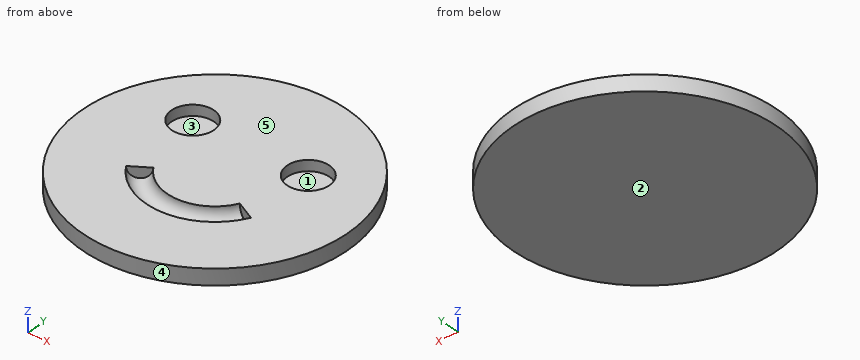
```python
from build123d import *

# Parameters (mm, degrees)
CYLINDER001_R         = 4
CYLINDER001_DEPTH     = 2
CYLINDER002_R         = 4
CYLINDER002_DEPTH     = 2
TORUS_R               = 2
TORUS_ANGLE           = 120
TORUS_PLACEMENT_ANGLE = 146
CYLINDER_R            = 25
CYLINDER_DEPTH        = 3


with BuildPart() as ull1:
    # Cylinder001 → Cylinder001 (new body)
    with BuildSketch(Plane(origin=(11, 8, 1), x_dir=(1, 0, 0), z_dir=(0, 0, 1))):
        Circle(CYLINDER001_R)
    extrude(amount=CYLINDER001_DEPTH)


with BuildPart() as ull2:
    # Cylinder002 → Cylinder002 (new body)
    with BuildSketch(Plane(origin=(-11, 8, 1), x_dir=(1, 0, 0), z_dir=(0, 0, 1))):
        Circle(CYLINDER002_R)
    extrude(amount=CYLINDER002_DEPTH)


with BuildPart() as boca:
    # Torus → Torus (revolve)
    with BuildSketch(Plane.XZ):
        with Locations((11, 0)):
            Circle(TORUS_R)
    revolve(axis=Axis((0, 0, 0), (0, 0, 1)), revolution_arc=TORUS_ANGLE)


with BuildPart() as boca_1:
    # Torus placement: moved
    add(boca.part.moved(Location((0, 0, 3))).rotate(Axis((0, 0, 3), (0, 0, -1)), TORUS_PLACEMENT_ANGLE))


with BuildPart() as cut002:
    # Cylinder → Cylinder (new body)
    with BuildSketch(Plane.XY):
        Circle(CYLINDER_R)
    extrude(amount=CYLINDER_DEPTH)

    # Cut: cut boca
    add(boca_1.part, mode=Mode.SUBTRACT)

    # Cut001: cut ull2
    add(ull2.part, mode=Mode.SUBTRACT)

    # Cut002: cut ull1
    add(ull1.part, mode=Mode.SUBTRACT)


solid = cut002.part
```
Could you check a few things on this model? Use its own coordinates, in mm. Face numbers are marked on the shaded views. A direction names the side the tool comes from. Round coordinates to 2 decimals unless told otherwise and drop trailing zeros. Loops run counter-clockwise (first coordinate to the right, second up) from the corner with the lowest first, then second, coordinate; pieces in that order, holes last.
Q1. I want a section at B-B (x = 0). Write out the boundary of the cut face in (y, z).
Q2. For P1, Ø1, axis at x = 13, z = 1.5, coming from the -Y side, with a flat end and sliding along its axis, tell me the tip position at first contact or that it passes through.
Q3. I want a section at A-A (z = 1.8). Write out the boundary of the cut face in (x, y), and give its area (3 significant figures).
Q4. On a 3-axis mill with a long thin cutter (end or side, diameter ignored), from which of +Z, -Z, +X, -X, +Y, -Y can I reach the whole of each face in a straight line? I mean the marked faces 1 and 2. Say none if no direction works.
Q5. Thinking about a two-plate mould opening in X: for the marked faces 3, 4 and 5, which applies, pulls with the +X half, pulls with the -X half, needs draft (parallel to the pull), parting line crosses it, or undercut?
Q6. Please list where these lines run through material, in increasing order: L1, parallel to X at y = 10.5, z = 1.95; L2, parallel to X at y = -20, z = 2.1; L3, parallel to Y at x = -11, z = 1.4.
Q7. I want a section at C-C (y = -15). Write out the boundary of the cut face in (x, z).
Q8. I want a section at D-D (y = 8). Write out the boundary of the cut face in (x, z).
Answer below:
1. outline: (-25, 0) - (25, 0) - (25, 3) - (-9, 3) arc R2 cw to (-13, 3) - (-25, 3) - close
2. P1: stops at y = -21.65
3. outline: circle Ø50 at (0, 0); hole circle Ø8 at (-11, 8); hole (-10.45, -7.05) arc R12.6 ccw to (11.32, -5.52) - (8.45, -4.12) arc R9.4 cw to (-7.79, -5.26) - close; hole circle Ø8 at (11, 8)
3. area: 1,790 mm2
4. face 1: +Z
4. face 2: -Z, +X, -X, +Y, -Y
5. face 3: undercut
5. face 4: parting line crosses it
5. face 5: needs draft
6. L1: x = -22.69 to -14.12, -7.88 to 7.88, 14.12 to 22.69
6. L2: x = -15 to 15
6. L3: y = -22.45 to 4, 12 to 22.45
7. outline: (-20, 0) - (20, 0) - (20, 3) - (-20, 3) - close
8. outline: (-23.69, 0) - (23.69, 0) - (23.69, 3) - (15, 3) - (15, 1) - (7, 1) - (7, 3) - (-7, 3) - (-7, 1) - (-15, 1) - (-15, 3) - (-23.69, 3) - close
